The listing builds one solid part. Answer for the finished solid, in the listing's coordinates (mm). A direction names the side the tool comes from. Coordinates: 2 decimals unless noted, no trailing zeros. Order: outer loops, then holes, each group sorted by start corner. A loop starts at its lowest first (then second) coordinate and runs counter-clockwise, first axis right, second up. Notation, with made-up numbers: (24.5, 4) -> (56.5, 4) arc R25 cw to (56.5, 32) -> close; hole circle Ø1 at (74, 52.25). An arc over 180 degrees is marked (long way). Return JSON: item names as keys, results as strings.
from build123d import *

# Parameters (mm, degrees)
SKETCH1_W           = 19.05
SKETCH1_H           = 25.4
BOSS_EXTRUDE1_DEPTH = 3.175
SKETCH2_R           = 3.175
BOSS_EXTRUDE2_DEPTH = 7.5125
SKETCH3_R           = 0.79375
CUT_EXTRUDE1_DEPTH  = 3.175
SKETCH4_R           = 7.9375
SKETCH4_R_2         = 6.35
BOSS_EXTRUDE3_DEPTH = 1


with BuildPart() as part:
    # Sketch1 → Boss-Extrude1 (new body)
    with BuildSketch(Plane(origin=(0, 0, 0), x_dir=(1, 0, 0), z_dir=(0, 1, 0))):
        with Locations((9.525, 12.7)):
            Rectangle(SKETCH1_W, SKETCH1_H)
    extrude(amount=BOSS_EXTRUDE1_DEPTH)

    # Sketch2 → Boss-Extrude2 (add)
    with BuildSketch(Plane(origin=(0, 3.175, 0), x_dir=(1, 0, 0), z_dir=(0, 1, 0))):
        with Locations((9.525, 12.7)):
            Circle(SKETCH2_R)
    extrude(amount=BOSS_EXTRUDE2_DEPTH)

    # Sketch3 → Cut-Extrude1 (cut)
    with BuildSketch(Plane(origin=(0, 3.175, 0), x_dir=(1, 0, 0), z_dir=(0, 1, 0))):
        with Locations((3.175, 22.225)):
            Circle(SKETCH3_R)
        with Locations((15.875, 22.225)):
            Circle(SKETCH3_R)
        with Locations((15.875, 3.175)):
            Circle(SKETCH3_R)
        with Locations((3.175, 3.175)):
            Circle(SKETCH3_R)
    extrude(amount=-CUT_EXTRUDE1_DEPTH, mode=Mode.SUBTRACT)

    # Sketch4 → Boss-Extrude3 (add)
    with BuildSketch(Plane(origin=(0, 3.175, 0), x_dir=(1, 0, 0), z_dir=(0, 1, 0))):
        with Locations((9.525, 12.7)):
            Circle(SKETCH4_R)
        with Locations((9.525, 12.7)):
            Circle(SKETCH4_R_2, mode=Mode.SUBTRACT)
    extrude(amount=BOSS_EXTRUDE3_DEPTH)


solid = part.part
1. The part is cut by section D-D on x = 7. Give the vertices of the cut face in (y, z) (1 decimal).
Answer block:
{"outline": "(0, -25.4) -> (3.2, -25.4) -> (3.2, -20.2) -> (4.2, -20.2) -> (4.2, -18.5) -> (3.2, -18.5) -> (3.2, -14.6) -> (10.7, -14.6) -> (10.7, -10.8) -> (3.2, -10.8) -> (3.2, -6.9) -> (4.2, -6.9) -> (4.2, -5.2) -> (3.2, -5.2) -> (3.2, 0) -> (0, 0) -> close"}
2. For faces 5 (the face through (12, 4.175, -19)), 6 (the face through (3, 1.61, -21.45)), determine the directions among +Z, -Z, +X, -X, +Y, -Y from which every point of the face is accessible in a straight line to the end or side of a thin tool.
Answer block:
{"face 5": "+Y", "face 6": "+Y, -Y"}
3. Consider line 1 (Y direction, x = 16.25, z = -20.25) (3 decimals); line 2 (Y direction, x = 13, z = -6.75) (3 decimals); line 3 (Z direction, x = 2.25, y = 3.5). Determine where each line is inside the solid, lowest interval first. Write a range as from..to.
Answer block:
{"line 1": "y = 0..3.175", "line 2": "y = 0..4.175", "line 3": "z = -15.87..-9.53"}
4. This flat-tipped pin is pushed along its axis until it touches: pin 1 Ø1 at (x, z) = (3.175, -22.225) entering from -Y. Where does it stop, or does it pass through?
Answer block:
{"pin 1": "passes through"}
5. The part is cut by section A-A on y = 3.5. Give the number of separate pieces and of enclosed holes in the cut face, and give its area (3 significant figures).
Answer block:
{"separate pieces": "2", "enclosed holes": "1", "area": "103 mm2"}
6. Determine the mould class of faces 1 (the face through (12.939, 3.668, -18.054)), 2 (the face through (9, 2, -25.4)), 3 (the face through (0, 2, -13)), 4 (the face through (9, 2, 0)) for opening direction Z: pulls with the +Z half, pulls with the -Z half, needs draft (parallel to the pull), parting line crosses it, or undercut.
Answer block:
{"face 1": "undercut", "face 2": "pulls with the -Z half", "face 3": "needs draft", "face 4": "pulls with the +Z half"}
